CAD build for the part. Positions are in the model's coordinates, mm. A direction names the side the tool comes from. Coordinates: 2 decimals unless noted, no trailing zeros. Write each loop counter-clockwise with the first axis right and the second up, starting at its lowest first coordinate (ties: lowest second). Pieces come first, ordered by that corner, then holes. Notation, with made-up numbers: (8.5, -34.5) - (66.5, -34.5) arc R32 ccw to (66.5, -2.5) - close; hole circle Ø11 at (-38, -17.75). An arc over 180 degrees is marked (long way). Answer in a Markdown table with one row per item. Add a question column.
Q1. 3-axis set-ups, long thin cutter, end or side, ignore diameter. For faces 1 (the flat face through (27.05, 6, 2)), 2 (the flat face through (41, 34, 2.5)), 3 (the flat face through (18.9, 22.3, 3)): which of +Z, -Z, +X, -X, +Y, -Y reach the whole face in a straight line?
Q2. Band-saw the part on B-B (y = 21). List the corners of the cut face in (x, z).
Q3. Pin check, flat tips, straight feed: pin 1 (1.9 mm diameter, centred on x = 20, y = 21, fed in from -Z); pin 2 (1.4 mm diameter, centred on x = 28.5, y = 33.5, fed in from -Z). Stop position of each tip, or through.
Q4. Two-plate mould, pull along Y, no slides. Class faces 4 (the flat face through (60, 23.85, 6)), 5 (the cylindrical face through (61.802, 0.713, 2.218)), 6 (the flat face through (18.95, 6, 2)): +Y half, -Y half, draft (parallel to the pull), parting line (faces both ways), or undercut.
Q5. Band-saw the part on A-A (x = 40). List the corners of the cut face in (y, z).
Q6. Drill centre lines: line 1 along Y through (x, z) = (23, 6.85); line 2 along X through (y, z) = (9.5, 2.5); line 3 along X through (y, z) = (19, 2.75). Where is each one in solid material? Low to high. Write a range as from..to.
Q7. Band-saw the part on C-C (z = 6.5). State how many separate pieces and enclosed holes the cut face has, and give its area (3 significant figures).
Q8. Band-saw the part on D-D (x = 48). List the corners of the cut face in (y, z).
```python
from build123d import *

# Parameters (mm, degrees)
SKETCH_2_W           = 80
SKETCH_2_H           = 35
SKETCH_2_R           = 4.05
EXTRUDE_1_DEPTH      = 8
SKETCH_3_R           = 2.55
CUT_EXTRUDE_1_DEPTH  = 88.686943156
CUT_EXTRUDE_2_DEPTH  = 88.686943156
SKETCH_5_R           = 1.55
CUT_EXTRUDE_3_DEPTH  = 88.686943156
CUT_EXTRUDE_4_DEPTH  = 4.5
CUT_EXTRUDE_5_DEPTH  = 4.5
SKETCH_11_R          = 1.55
CUT_EXTRUDE_7_DEPTH  = 88.686943156
CUT_EXTRUDE_8_DEPTH  = 3
CUT_EXTRUDE_START    = -3
CUT_EXTRUDE_9_DEPTH  = 3
CUT_EXTRUDE_11_DEPTH = 1


with BuildPart() as part:
    # 草图2 → 凸台-拉伸1 (new body)
    with BuildSketch(Plane.XY):
        with Locations((40, 17.5)):
            Rectangle(SKETCH_2_W, SKETCH_2_H)
        with Locations((7, 8)):
            Circle(SKETCH_2_R, mode=Mode.SUBTRACT)
        with Locations((40, 10)):
            Circle(SKETCH_2_R, mode=Mode.SUBTRACT)
        with Locations((73, 8)):
            Circle(SKETCH_2_R, mode=Mode.SUBTRACT)
    extrude(amount=EXTRUDE_1_DEPTH)

    # 草图3 → 切除-拉伸1 (cut, through all)
    with BuildSketch(Plane.XY.offset(8)):
        with Locations((23, 8)):
            Circle(SKETCH_3_R)
        with Locations((57, 8)):
            Circle(SKETCH_3_R)
    extrude(amount=-CUT_EXTRUDE_1_DEPTH, mode=Mode.SUBTRACT)

    # 草图4 → 切除-拉伸2 (cut, through all)
    with BuildSketch(Plane(origin=(80, 0, 0), x_dir=(0, 0, -1), z_dir=(1, 0, 0))):
        Polygon((-1.5, 33.2), (-2.5, 33.2), (-2.5, 35), (0, 35), (0, 29.8), (-1.5, 29.8), align=None)
    extrude(amount=-CUT_EXTRUDE_2_DEPTH, mode=Mode.SUBTRACT)

    # 草图5 → 切除-拉伸3 (cut, through all)
    with BuildSketch(Plane.XY.offset(8)):
        with Locations((48, 10)):
            Circle(SKETCH_5_R)
        with Locations((32, 10)):
            Circle(SKETCH_5_R)
    extrude(amount=-CUT_EXTRUDE_3_DEPTH, mode=Mode.SUBTRACT)

    # 草图7 → 切除-拉伸4 (cut)
    with BuildSketch(Plane(origin=(0, 0, 0), x_dir=(-1, 0, 0), z_dir=(0, 0, -1))):
        with BuildLine():
            Line((-27.05, 10), (-27.05, 2.5))
            ThreePointArc((-27.05, 2.5), (-27.782233047, 0.732233047), (-29.55, 0))
            Line((-29.55, 0), (-16.45, 0))
            ThreePointArc((-16.45, 0), (-18.217766953, 0.732233047), (-18.95, 2.5))
            Line((-18.95, 2.5), (-18.95, 10))
            ThreePointArc((-18.95, 10), (-23, 14.05), (-27.05, 10))
        make_face()
        with BuildLine():
            Line((-61.05, 2.5), (-61.05, 10))
            ThreePointArc((-61.05, 10), (-57, 14.05), (-52.95, 10))
            Line((-52.95, 10), (-52.95, 2.5))
            ThreePointArc((-52.95, 2.5), (-52.217766953, 0.732233047), (-50.45, 0))
            Line((-50.45, 0), (-63.55, 0))
            ThreePointArc((-63.55, 0), (-61.782233047, 0.732233047), (-61.05, 2.5))
        make_face()
    extrude(amount=-CUT_EXTRUDE_4_DEPTH, mode=Mode.SUBTRACT)

    # 草图8 → 切除-拉伸5 (cut)
    with BuildSketch(Plane(origin=(0, 0, 0), x_dir=(-1, 0, 0), z_dir=(0, 0, -1))):
        with BuildLine():
            Line((-30.5, 12.85), (-49.5, 12.85))
            ThreePointArc((-49.5, 12.85), (-52.35, 10), (-49.5, 7.15))
            Line((-49.5, 7.15), (-30.5, 7.15))
            ThreePointArc((-30.5, 7.15), (-27.65, 10), (-30.5, 12.85))
        make_face()
    extrude(amount=-CUT_EXTRUDE_5_DEPTH, mode=Mode.SUBTRACT)

    # 草图11 → 切除-拉伸7 (cut, through all)
    with BuildSketch(Plane(origin=(0, 0, 0), x_dir=(-1, 0, 0), z_dir=(0, 0, -1))):
        with Locations((-60, 21)):
            Circle(SKETCH_11_R)
        with Locations((-20, 21)):
            Circle(SKETCH_11_R)
    extrude(amount=-CUT_EXTRUDE_7_DEPTH, mode=Mode.SUBTRACT)

    # 草图12 → 切除-拉伸8 (cut)
    with BuildSketch(Plane(origin=(0, 0, 0), x_dir=(-1, 0, 0), z_dir=(0, 0, -1))):
        with BuildLine():
            Line((-62.5, 18.15), (-57.5, 18.15))
            ThreePointArc((-57.5, 18.15), (-54.65, 21), (-57.5, 23.85))
            Line((-57.5, 23.85), (-62.5, 23.85))
            ThreePointArc((-62.5, 23.85), (-65.35, 21), (-62.5, 18.15))
        make_face()
        with BuildLine():
            Line((-17.5, 23.85), (-22.5, 23.85))
            ThreePointArc((-22.5, 23.85), (-25.35, 21), (-22.5, 18.15))
            Line((-22.5, 18.15), (-17.5, 18.15))
            ThreePointArc((-17.5, 18.15), (-14.65, 21), (-17.5, 23.85))
        make_face()
    extrude(amount=-CUT_EXTRUDE_8_DEPTH, mode=Mode.SUBTRACT)

    # 草图15 → 切除-拉伸9 (cut)
    with BuildSketch(Plane.XY.offset(8).offset(CUT_EXTRUDE_START)):
        with BuildLine():
            Line((57.5, 18.15), (62.5, 18.15))
            ThreePointArc((62.5, 18.15), (65.35, 21), (62.5, 23.85))
            Line((62.5, 23.85), (57.5, 23.85))
            ThreePointArc((57.5, 23.85), (54.65, 21), (57.5, 18.15))
        make_face()
        with BuildLine():
            Line((22.5, 23.85), (17.5, 23.85))
            ThreePointArc((17.5, 23.85), (14.65, 21), (17.5, 18.15))
            Line((17.5, 18.15), (22.5, 18.15))
            ThreePointArc((22.5, 18.15), (25.35, 21), (22.5, 23.85))
        make_face()
    extrude(amount=CUT_EXTRUDE_9_DEPTH, mode=Mode.SUBTRACT)

    # 草图19 → 切除-拉伸11 (cut, symmetric)
    with BuildSketch(Plane(origin=(0, 0, 2.5), x_dir=(-1, 0, 0), z_dir=(0, 0, -1))):
        with BuildLine():
            Line((-25, 35), (-55.247938178, 35))
            Line((-55.247938178, 35), (-55.247938178, 34.2))
            ThreePointArc((-55.247938178, 34.2), (-54.747938178, 33.7), (-54.247938178, 34.2))
            Line((-54.247938178, 34.2), (-26, 34.2))
            ThreePointArc((-26, 34.2), (-25.5, 33.7), (-25, 34.2))
            Line((-25, 34.2), (-25, 35))
        make_face()
    extrude(amount=CUT_EXTRUDE_11_DEPTH, both=True, mode=Mode.SUBTRACT)


solid = part.part
```
Checked values:
| question | item | result |
|---|---|---|
| 1 | face 1 | -Z, -Y |
| 1 | face 2 | -Z, +X, -X, +Y |
| 1 | face 3 | -Z |
| 2 | outline | (0, 0) - (14.65, 0) - (14.65, 3) - (18.45, 3) - (18.45, 5) - (14.65, 5) - (14.65, 8) - (0, 8) - close; (21.55, 3) - (25.35, 3) - (25.35, 0) - (54.65, 0) - (54.65, 3) - (58.45, 3) - (58.45, 5) - (54.65, 5) - (54.65, 8) - (25.35, 8) - (25.35, 5) - (21.55, 5) - close; (61.55, 3) - (65.35, 3) - (65.35, 0) - (80, 0) - (80, 8) - (65.35, 8) - (65.35, 5) - (61.55, 5) - close |
| 3 | pin 1 | passes through |
| 3 | pin 2 | stops at z = 1.5 |
| 4 | face 4 | undercut |
| 4 | face 5 | -Y half |
| 4 | face 6 | draft |
| 5 | outline | (0, 0) - (5.95, 0) - (5.95, 8) - (0, 8) - close; (14.05, 0) - (29.8, 0) - (29.8, 1.5) - (33.2, 1.5) - (33.2, 2.5) - (34.2, 2.5) - (34.2, 3.5) - (35, 3.5) - (35, 8) - (14.05, 8) - close |
| 6 | line 1 | y = 0..5.45, 10.55..18.19, 23.81..35 |
| 6 | line 2 | x = 0..3.24, 10.76..18.95, 27.05..27.69, 52.31..52.95, 61.05..69.24, 76.76..80 |
| 6 | line 3 | x = 0..15.47, 24.53..55.47, 64.53..80 |
| 7 | separate pieces | 1 |
| 7 | enclosed holes | 9 |
| 7 | area | 2,480 mm² |
| 8 | outline | (0, 0) - (7.15, 0) - (7.15, 4.5) - (8.45, 4.5) - (8.45, 8) - (0, 8) - close; (11.55, 4.5) - (12.85, 4.5) - (12.85, 0) - (29.8, 0) - (29.8, 1.5) - (33.2, 1.5) - (33.2, 2.5) - (34.2, 2.5) - (34.2, 3.5) - (35, 3.5) - (35, 8) - (11.55, 8) - close |
